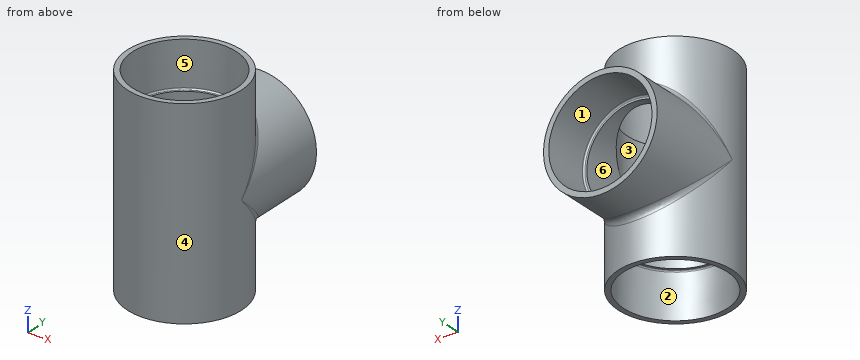
```python
from build123d import *

# Parameters (mm, degrees)
BOSS_EXTRUDE1_REACH      = 178.609
BOSS_EXTRUDE1_END_RADIUS = 63.896875
SKETCH2_R                = 63.896875
CUT_EXTRUDE1_REACH       = 127.809
CUT_EXTRUDE1_END_RADIUS  = 53.34
SKETCH4_R                = 53.34
FILLET1_R                = 1.5875
FILLET2_R                = 6.35


with BuildPart() as part:
    # Sketch1 → Revolve1 (revolve)
    with BuildSketch(Plane(origin=(0, 0, 0), x_dir=(0, 0, -1), z_dir=(1, 0, 0)), mode=Mode.PRIVATE) as revolve1_sk:
        Polygon((-112.7125, 63.896875), (112.7125, 63.896875), (112.7125, 58.036717298), (61.9125, 57.15), (61.9125, 53.34), (-61.9125, 53.34), (-61.9125, 57.15), (-112.7125, 58.036717298), align=None)
    revolve(revolve1_sk.sketch.rotate(Axis((0, 0, 168.705111385), (0, 0, -1)), 90), axis=Axis((0, 0, 168.705111385), (0, 0, -1)))  # turned: the seam where the file's is

    # Boss-Extrude1: up to this cylinder (the profile starts outside it)
    boss_extrude1_end = Plane(origin=(0, 0, 0), z_dir=(0, 0, 1)) * Cylinder(BOSS_EXTRUDE1_END_RADIUS, 486.01175, mode=Mode.PRIVATE)
    # Sketch2 → Boss-Extrude1 (add, up to the surface)
    with BuildSketch(Plane(origin=(0, 112.7125, 0), x_dir=(1, 0, 0), z_dir=(0, 1, 0)), mode=Mode.PRIVATE) as boss_extrude1_sk1:
        with Locations(Location((0, 0, 0), (0, 0, 270))):  # turned: the seam where the file's is
            Circle(SKETCH2_R)
    boss_extrude1_tool1 = extrude(boss_extrude1_sk1.sketch, amount=-BOSS_EXTRUDE1_REACH, mode=Mode.PRIVATE) - boss_extrude1_end
    add(boss_extrude1_tool1.solids().sort_by_distance((0, 112.7125, 0))[0])

    # Sketch3 → Cut-Revolve1 (revolve, cut)
    with BuildSketch(Plane(origin=(0, 0, 0), x_dir=(0, 0, -1), z_dir=(1, 0, 0))):
        Polygon((-58.036717298, 112.7125), (-57.15, 61.9125), (0, 61.9125), (0, 112.7125), align=None)
    revolve(axis=Axis((0, 0, 0), (0, 1, 0)), mode=Mode.SUBTRACT)

    # Cut-Extrude1: up to this cylinder (the profile starts outside it)
    cut_extrude1_end = Plane(origin=(0, 0, 0), z_dir=(0, 0, 1)) * Cylinder(CUT_EXTRUDE1_END_RADIUS, 363.298, mode=Mode.PRIVATE)
    # Sketch4 → Cut-Extrude1 (cut, up to the surface)
    with BuildSketch(Plane(origin=(0, 61.9125, 0), x_dir=(1, 0, 0), z_dir=(0, 1, 0)), mode=Mode.PRIVATE) as cut_extrude1_sk1:
        with Locations(Location((0, 0, 0), (0, 0, 270))):  # turned: the seam where the file's is
            Circle(SKETCH4_R)
    cut_extrude1_tool1 = extrude(cut_extrude1_sk1.sketch, amount=-CUT_EXTRUDE1_REACH, mode=Mode.PRIVATE) - cut_extrude1_end
    add(cut_extrude1_tool1.solids().sort_by_distance((0, 61.9125, 0))[0], mode=Mode.SUBTRACT)

    # Fillet1
    fillet1_edges = [part.edges().sort_by_distance(p)[0] for p in [
        (0, 61.9125, -57.15),
        (-57.15, 0, 61.9125),
        (-57.15, 0, -61.9125),
    ]]
    fillet(fillet1_edges, radius=FILLET1_R)

    # Fillet2
    fillet2_edges = [part.edges().sort_by_distance(p)[0] for p in [
        (48.772230172, 41.280506281, 41.280506281),
        (-48.772230172, 41.280506281, -41.280506281),
    ]]
    fillet(fillet2_edges, radius=FILLET2_R)


solid = part.part
```
The model under review builds one solid part; all positions refer to its coordinate system, in mm. Face numbers are marked on the shaded views. A direction names the side the tool comes from. Coordinates: 2 decimals unless noted, no trailing zeros. Write each loop counter-clockwise with the first axis right and the second up, starting at its lowest first coordinate (ties: lowest second). Pieces come first, ordered by that corner, then holes. Notation, with made-up numbers: (36.5, 69.25) - (85.5, 69.25) arc R15 ccw to (85.5, 73.25) - close; hole circle Ø4 at (38, -11). An arc over 180 degrees is marked (long way). Answer in a Markdown table with one row per item. Add a question column.
Q1. Clearance check with flat-ended pins moving along their axes: pin 1 (12 mm diameter, centred on x = -31, z = 37.5, fed in from +Y); pin 2 (12 mm diameter, centred on x = 49, z = 81.5, fed in from -Y); pin 3 (1 mm diameter, centred on y = -16.5, z = 51.5, fed in from -X); pin 4 (6 mm diameter, centred on x = -43, z = 37.5, fed in from +Y). State where each tip first meets the part, or that it passes through.
Q2. Consider section A-A on x = 45.5. Give the number of separate pieces and of enclosed holes in the cut face, then the cut area to 3 significant figures.
Q3. Consider section C-C on y = 90. Give the boundary of the cut face in (x, z), then the cut area to 3 significant figures.
Q4. For the marked faces 5 and 6, list the 3-axis set-ups (+Z, -Z, +X, -X, +Y, -Y) from which the entire face can be reached by the end or side of a thin tool; tool diameter is ignored.
Q5. Consider section B-B on z = 80.5. Give the boundary of the cut face in (x, y).
Q6. To check wall thickness, follow line 1 along X through (y, z) = (28, 0); line 2 along Y through (x, z) = (0, 11); line 3 along X through (y, z) = (36, 70). State the ranges of each line that lie inside material, in increasing order. Write a range as from..to.
Q7. Draft analysis for pull direction Y (two halves, no side actions). For the marked faces 1, 2, 3 and 4, state which applies: +Y half, -Y half, draft (parallel to the pull), parting line (faces both ways), or undercut.
Answers below:
| question | item | result |
|---|---|---|
| 1 | pin 1 | y = 61.91 |
| 1 | pin 2 | y = -47.26 |
| 1 | pin 3 | x = -61.86 |
| 1 | pin 4 | y = 112.71 |
| 2 | separate pieces | 3 |
| 2 | enclosed holes | 0 |
| 2 | area | 6,770 mm² |
| 3 | outline | circle Ø127.79 at (0, 0); hole circle Ø115.28 at (0, 0) |
| 3 | area | 2,390 mm² |
| 4 | face 5 | +Z |
| 4 | face 6 | +Y |
| 5 | outline | circle Ø127.79 at (0, 0); hole circle Ø114.95 at (0, 0) |
| 6 | line 1 | -63.9..-53.34, 53.34..63.9 |
| 6 | line 2 | -63.9..-53.34 |
| 6 | line 3 | -52.79..-44.57, 44.57..52.79 |
| 7 | face 1 | +Y half |
| 7 | face 2 | undercut |
| 7 | face 3 | undercut |
| 7 | face 4 | parting line |
